CAD build for the part. Positions are in the model's coordinates, mm. A direction names the side the tool comes from. Give positions to 0.01 mm unless a question says otherwise; leave off trailing zeros. Loops run counter-clockwise (first coordinate to the right, second up) from the corner with the lowest first, then second, coordinate; pieces in that order, holes last.
```python
from build123d import *

# Parameters (mm, degrees)
F0_R     = 22.5
F0_R_2   = 18
F1_DEPTH = 3
F2_DEPTH = 30
F3_R     = 1
F4_R     = 2.5
F5_DEPTH = 25
F6_R     = 1


with BuildPart() as f1:
    # F0 (on Front) → F1 (new body)
    with BuildSketch(Plane.XZ):
        Circle(F0_R)
        Circle(F0_R_2, mode=Mode.SUBTRACT)
        Circle(F0_R_2)
    extrude(amount=F1_DEPTH)

    # F0 (on Front) → F2 (join)
    with BuildSketch(Plane.XZ):
        Circle(F0_R)
        Circle(F0_R_2, mode=Mode.SUBTRACT)
    extrude(amount=F2_DEPTH)

    # F3
    f3_edges = [f1.edges().sort_by_distance(p)[0] for p in [
        (-18, -3, 0),
        (-22.5, -30, 0),
        (-22.5, 0, 0),
    ]]
    fillet(f3_edges, radius=F3_R)

    # F4 (on face) → F5 (cut)
    with BuildSketch(Plane(origin=(0, 0, 0), x_dir=(-1, 0, 0), z_dir=(0, 1, 0))):
        Circle(F4_R)
    extrude(amount=-F5_DEPTH, mode=Mode.SUBTRACT)

    # F6
    f6_edges = [f1.edges().sort_by_distance(p)[0] for p in [
        (2.5, -3, 0),
        (2.5, 0, 0),
    ]]
    fillet(f6_edges, radius=F6_R)


solid = f1.part
```
1. Probe line 1 along Z through (x, y) = (0.5, -19.5); line 2 along X through (y, z) = (-10.25, 8); line 3 along Z through (x, y) = (-7, -15.5). List the from-to ranges inside material, lowest first.
Responses:
line 1: z = -22.49 to -17.99, 17.99 to 22.49
line 2: x = -21.03 to -16.12, 16.12 to 21.03
line 3: z = -21.38 to -16.58, 16.58 to 21.38
2. Saw through at B-B, the plane z = 0. List the corners of the cut face in (x, y), and give its area (3 significant figures).
Responses:
outline: (-22.5, -29) arc R1 ccw to (-21.5, -30) - (-18, -30) - (-18, -4) arc R1 cw to (-17, -3) - (-3.5, -3) arc R1 ccw to (-2.5, -2) - (-2.5, -1) arc R1 ccw to (-3.5, 0) - (-21.5, 0) arc R1 ccw to (-22.5, -1) - close; (2.5, -2) arc R1 ccw to (3.5, -3) - (17, -3) arc R1 cw to (18, -4) - (18, -30) - (21.5, -30) arc R1 ccw to (22.5, -29) - (22.5, -1) arc R1 ccw to (21.5, 0) - (3.5, 0) arc R1 ccw to (2.5, -1) - close
area: 362 mm2
3. Saw through at C-C, the plane y = -6. List the corners of the cut face in (x, z).
Responses:
outline: circle Ø45 at (0, 0); hole circle Ø36 at (0, 0)
4. Drop flat-ended pins along their axis: pin 1 (12 mm diameter, centred on y = -26.5, z = -14, fed in from +X); pin 2 (21.5 mm diameter, centred on x = 0, z = 0, fed in from +Y); pin 3 (6 mm diameter, centred on y = -27, z = -10, fed in from +X); pin 4 (1.5 mm diameter, centred on x = -3, y = -26, fed in from +Z). Give the stop position or say it passes through.
Responses:
pin 1: stops at x = 21.03
pin 2: stops at y = 0
pin 3: stops at x = 21.38
pin 4: stops at z = 22.39
5. Pull direction X, two halves, no side cores. Call faces 3 (the face through (-13, -30, -13)), 4 (the face through (10.382, -14.804, -19.961)), 5 (the face through (-2.343, -16.818, 17.847)): released by +X, released by -X, zero draft, split by the parting line, or undercut.
Responses:
face 3: zero draft
face 4: split by the parting line
face 5: undercut
6. Tool access for faces 1 (the face through (4, -3, 0)), 2 (the face through (0.54, -1.49, -2.44)): list every direction of +Z, -Z, +X, -X, +Y, -Y with a clear straight run to the whole face (end or side of a thin tool).
Responses:
face 1: -Y
face 2: +Y, -Y
7. Saw through at A-A, the plane x = 0. List the corners of the cut face in (y, z).
Responses:
outline: (-30, -21.5) arc R1 ccw to (-29, -22.5) - (-1, -22.5) arc R1 ccw to (0, -21.5) - (0, -3.5) arc R1 ccw to (-1, -2.5) - (-2, -2.5) arc R1 ccw to (-3, -3.5) - (-3, -17) arc R1 cw to (-4, -18) - (-30, -18) - close; (-30, 18) - (-4, 18) arc R1 cw to (-3, 17) - (-3, 3.5) arc R1 ccw to (-2, 2.5) - (-1, 2.5) arc R1 ccw to (0, 3.5) - (0, 21.5) arc R1 ccw to (-1, 22.5) - (-29, 22.5) arc R1 ccw to (-30, 21.5) - close
